Here's how the part is built. I have some questions about the finished solid (model axes, mm). Face numbers are marked on the shaded views. Coordinates: 2 decimals unless noted, no trailing zeros. Loops run counter-clockwise (first coordinate to the right, second up) from the corner with the lowest first, then second, coordinate; pieces in that order, holes last.
from build123d import *

# Parameters (mm, degrees)
SKETCH1_W           = 56
SKETCH1_H           = 100
BOSS_EXTRUDE1_DEPTH = 7
SKETCH2_R           = 14.275
CUT_EXTRUDE1_DEPTH  = 8
SKETCH3_R           = 11
CUT_EXTRUDE2_DEPTH  = 10
SKETCH4_R           = 2.5
CUT_EXTRUDE3_DEPTH  = 8
FILLET1_R           = 10


with BuildPart() as part:
    # Sketch1 → Boss-Extrude1 (new body)
    with BuildSketch(Plane.XY):
        with Locations((28, 50)):
            Rectangle(SKETCH1_W, SKETCH1_H)
    extrude(amount=BOSS_EXTRUDE1_DEPTH)

    # Sketch2 → Cut-Extrude1 (cut, through all)
    with BuildSketch(Plane.XY.offset(7)):
        with Locations((28, 28)):
            Circle(SKETCH2_R)
        with BuildLine():
            Line((10.5, 30), (10.5, 8))
            ThreePointArc((10.5, 8), (8, 5.5), (5.5, 8))
            Line((5.5, 8), (5.5, 30))
            ThreePointArc((5.5, 30), (8, 32.5), (10.5, 30))
        make_face()
        with BuildLine():
            Line((50.5, 30), (50.5, 8))
            ThreePointArc((50.5, 8), (48, 5.5), (45.5, 8))
            Line((45.5, 8), (45.5, 30))
            ThreePointArc((45.5, 30), (48, 32.5), (50.5, 30))
        make_face()
    extrude(amount=-CUT_EXTRUDE1_DEPTH, mode=Mode.SUBTRACT)

    # Sketch3 → Cut-Extrude2 (cut)
    with BuildSketch(Plane(origin=(0, 0, 0), x_dir=(-1, 0, 0), z_dir=(0, 0, -1))):
        with Locations((-28, 68.5)):
            Circle(SKETCH3_R)
    extrude(amount=-CUT_EXTRUDE2_DEPTH, mode=Mode.SUBTRACT)

    # Sketch4 → Cut-Extrude3 (cut, through all)
    with BuildSketch(Plane(origin=(0, 0, 0), x_dir=(-1, 0, 0), z_dir=(0, 0, -1))):
        with Locations((-45.965981938, 86.45504088)):
            Circle(SKETCH4_R)
        with Locations((-28.007736497, 93.899998822)):
            Circle(SKETCH4_R)
        with Locations((-10.04495912, 86.465981938)):
            Circle(SKETCH4_R)
        with Locations((-45.95504088, 50.534018062)):
            Circle(SKETCH4_R)
        with Locations((-10.034018062, 50.54495912)):
            Circle(SKETCH4_R)
    extrude(amount=-CUT_EXTRUDE3_DEPTH, mode=Mode.SUBTRACT)

    # Fillet1
    fillet1_edges = [part.edges().sort_by_distance(p)[0] for p in [
        (56, 100, 3.5),
        (0, 100, 3.5),
    ]]
    fillet(fillet1_edges, radius=FILLET1_R)


solid = part.part
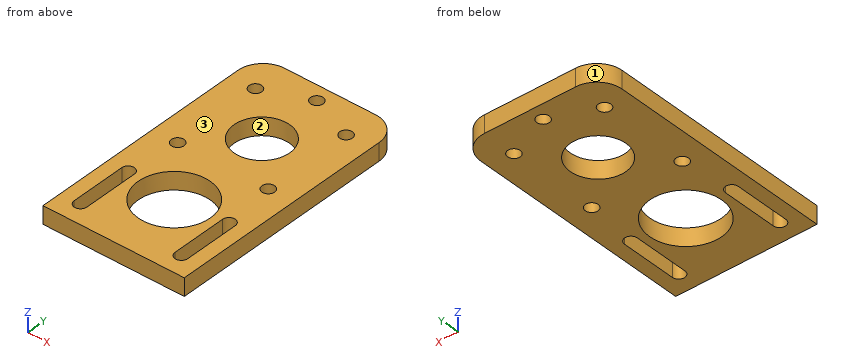
Q1. Will this pin go through, and if not, where does the flat tip stop? P1, Ø4.5, axis at x = 45.97, y = 86.46, coming from the +Z side.
Q2. Suppose I cut it at B-B on y = 61. Write out the boundary of the cut face in (x, z).
Q3. Suppose I cut it at C-C on z = 5.75. State how many separate pieces and enclosed holes the cut face has, and give its area (3 significant figures).
Q4. Suppose I cut it at A-A on y = 28. Write out the boundary of the cut face in (x, z) (3 decimals), and give its area (3 significant figures).
Q5. Please list where these lines run through material, in increasing order: probe 1 along X at (y, z) = (85, 1.5); probe 2 along Y at (x, z) = (23, 2.75); probe 3 along Y at (x, z) = (23.5, 0.75).
Q6. Suppose I cut it at D-D on x = 28. Write out the boundary of the cut face in (y, z) (3 decimals), and give its area (3 significant figures).
Q7. We'd pull the mould along X, two halves only. Please class the marked faces 1, 2 and 3: pulls with the +X half, pulls with the -X half, needs draft (parallel to the pull), parting line crosses it, or undercut.
Check values:
1. P1: passes through
2. outline: (0, 0) - (19.95, 0) - (19.95, 7) - (0, 7) - close; (36.05, 0) - (56, 0) - (56, 7) - (36.05, 7) - close
3. separate pieces: 1
3. enclosed holes: 9
3. area: 4,180 mm2
4. outline: (0, 0) - (5.5, 0) - (5.5, 7) - (0, 7) - close; (10.5, 0) - (13.725, 0) - (13.725, 7) - (10.5, 7) - close; (42.275, 0) - (45.5, 0) - (45.5, 7) - (42.275, 7) - close; (50.5, 0) - (56, 0) - (56, 7) - (50.5, 7) - close
4. area: 122 mm2
5. probe 1: x = 0 to 8.02, 12.07 to 43.93, 48 to 56
5. probe 2: y = 0 to 14.63, 41.37 to 58.7, 78.3 to 100
5. probe 3: y = 0 to 14.45, 41.55 to 58.46, 78.54 to 100
6. outline: (0, 0) - (13.725, 0) - (13.725, 7) - (0, 7) - close; (42.275, 0) - (57.5, 0) - (57.5, 7) - (42.275, 7) - close; (79.5, 0) - (91.4, 0) - (91.4, 7) - (79.5, 7) - close; (96.4, 0) - (100, 0) - (100, 7) - (96.4, 7) - close
6. area: 311 mm2
7. face 1: pulls with the -X half
7. face 2: undercut
7. face 3: needs draft
